Autodesk Inventor part; units mm, degrees
ref_plane "YZ Plane" through (0, 0, 0) normal (1, 0, 0) x (0, 1, 0)
ref_plane "XZ Plane" through (0, 0, 0) normal (0, 1, 0) x (-1, 0, 0)
ref_plane "XY Plane" through (0, 0, 0) normal (0, 0, 1) x (1, 0, 0)
sketch "Sketch1" plane through (0, 0, 0) normal (0, 1, 0) x (-1, 0, 0)
  line L0 (101.6, -101.6) -> (-101.6, -101.6)
  line L1 (-101.6, -101.6) -> (-101.6, 101.6)
  line L2 (-101.6, 101.6) -> (101.6, 101.6)
  line L3 (101.6, 101.6) -> (101.6, -101.6)
  line L4 (96.6, -96.6) -> (-96.6, -96.6)
  line L5 (-96.6, -96.6) -> (-96.6, 96.6)
  line L6 (-96.6, 96.6) -> (96.6, 96.6)
  line L7 (96.6, 96.6) -> (96.6, -96.6)
  line L8 (101.6, 101.6) -> (-40.4, 101.6)
  circle A0 centre (0, 0) radius 88.9
  line L9 (-40.4, 101.6) -> (-101.6, 40.4)
  line L10 (-45.4, 101.6) -> (-101.6, 45.4)
  line L11 (96.6, 96.6) -> (96.6, 101.6)
  line L12 (-45.4, 101.6) -> (-35.4, 101.6)
  line L13 (-35.4, 101.6) -> (-35.4, 96.6)
  line L14 (-35.4, 96.6) -> (-45.4, 96.6)
  line L15 (-45.4, 96.6) -> (-45.4, 101.6)
  line L16 (-101.6, 39.4) -> (-39.4, 101.6)
  line L17 (96.4, -96.4) -> (-96.4, -96.4)
  line L18 (-96.4, -96.4) -> (-96.4, 96.4)
  line L19 (-96.4, 96.4) -> (96.4, 96.4)
  line L20 (96.4, 96.4) -> (96.4, -96.4)
  circle A1 centre (0, 0) radius 90.9
  point P0 (96.6, 51.2168)
  point P1 (101.6, 40.4)
  point P2 (101.6, -40.4)
  point P3 (96.6, -51.2168)
  point P4 (-96.6, 45.4)
  point P5 (-45.4, 96.6)
  point P6 (-44.6, 96.4)
  point P7 (-96.4, 44.6)
  dimension "d0" = 203.2
  dimension "d1" = 203.2
  dimension "d2" = 101.6
  dimension "d3" = 101.6
  dimension "d4" = 5
  dimension "d5" = 5
  dimension "d6" = 5
  dimension "d7" = 5
  dimension "d8" = 142
  dimension "d9" = 61.2
  dimension "d10" = 177.8
  dimension "d11" = 5
  dimension "d12" = 5
  dimension "d13" = 10
  dimension "d14" = 1
  dimension "d15" = 0.2
  dimension "d16" = 0.2
  dimension "d17" = 0.2
  dimension "d18" = 0.2
  dimension "d64" = 181.8
extrude "Extrusion1" add sketch "Sketch1" along normal blind 4 contours L16 L19 L20 L17 L18
sketch "Sketch6" plane through (0, 4, 0) normal (0, 1, 0) x (1, 0, 0)
  line L0 (96.4, 96.4) -> (-96.4, 96.4)
  line L1 (96.4, 96.4) -> (88.4, 96.4)
  line L2 (88.4, 96.4) -> (88.4, -45.6)
  line L3 (88.4, -45.6) -> (96.4, -45.6)
  line L4 (96.4, -45.6) -> (96.4, 96.4)
  line L5 (96.4, -44.6) -> (96.4, 96.4)
  line L6 (88.4, -12) -> (96.4, -12)
  line L7 (96.4, -12) -> (96.4, 12)
  line L8 (96.4, 12) -> (88.4, 12)
  line L9 (88.4, 12) -> (88.4, -12)
  line L10 (0, 0) -> (96.4, 0)
  point P0 (96.4, -12)
  dimension "d58" = 8
  dimension "d59" = 142
  dimension "d62" = 12
  dimension "d63" = 12
extrude "Extrusion6" cut sketch "Sketch6" against normal blind 25.4 contours L4 L10 L2 L8 | L4 L6 L2 L10
sketch "Sketch8" plane through (0, 4, 0) normal (0, 1, 0) x (1, 0, 0)
  line L0 (-96.6, 96.6) -> (-96.6, -96.6)
  line L1 (96.6, 96.6) -> (-96.6, 96.6)
  line L2 (-96.6, 96.6) -> (96.6, 96.6)
  line L3 (96.6, -45.4) -> (45.4, -96.6)
  line L4 (96.6, 96.6) -> (96.6, -45.4)
  line L5 (96.6, -45.4) -> (45.4, -96.6)
  line L6 (45.4, -96.6) -> (-96.6, -96.6)
  line L7 (-96.6, -96.6) -> (-96.6, 96.6)
  line L8 (-96.6, 96.6) -> (-89.5289, 89.5289)
  circle A0 centre (-89.5289, 89.5289) radius 5
  circle A1 centre (-89.5289, 89.5289) radius 1.5
  line L9 (-89.5289, 84.5289) -> (-96.6, 84.5289)
  line L10 (-89.5289, 89.5289) -> (-89.5289, 84.5289)
  line L11 (-89.5289, 89.5289) -> (-84.5289, 89.5289)
  line L12 (-84.5289, 96.6) -> (-84.5289, 89.5289)
  line L13 (-96.6, -96.6) -> (-89.5289, -89.5289)
  line L14 (-96.6, -96.6) -> (-86.6, -96.6) construction
  circle A2 centre (-89.5289, -89.5289) radius 5
  circle A3 centre (-89.5289, -89.5289) radius 1.75
  line L15 (-89.5289, -89.5289) -> (-84.5289, -89.5289)
  line L16 (-84.5289, -96.6) -> (-84.5289, -89.5289)
  line L17 (-89.5289, -89.5289) -> (-89.5289, -84.5289)
  line L18 (-96.6, -84.5289) -> (-89.5289, -84.5289)
  line L19 (96.6, 96.6) -> (89.5289, 89.5289)
  circle A4 centre (89.5289, 89.5289) radius 5
  circle A5 centre (89.5289, 89.5289) radius 1.75
  line L20 (89.5289, 89.5289) -> (84.5289, 89.5289)
  line L21 (84.5289, 96.6) -> (84.5289, 89.5289)
  line L22 (89.5289, 89.5289) -> (89.5289, 84.5289)
  line L23 (96.6, 84.5289) -> (89.5289, 84.5289)
  line L24 (96.6, -43.114) -> (96.6, 96.6)
  line L25 (-96.6, -96.6) -> (43.1178, -96.6)
  line L26 (28.9914, 5.6569) -> (-5.6569, -28.9914)
  line L27 (25.4, -25.4) -> (101.6, -25.4)
  line L28 (101.6, -88.9) -> (101.6, 101.6)
  line L29 (25.4, -25.4) -> (25.4, -101.6)
  line L30 (43.1178, -101.6) -> (-101.6, -101.6)
  line L31 (96.6, -25.4) -> (86.6, -25.4)
  circle A6 centre (86.6, -25.4) radius 5
  circle A7 centre (86.6, -25.4) radius 1.75
  line L32 (25.4, -96.6) -> (25.4, -86.6)
  circle A8 centre (25.4, -86.6) radius 5
  circle A9 centre (25.4, -86.6) radius 1.75
  line L33 (44.6, -96.4) -> (96.4, -44.6)
  circle A10 centre (68.7322, -68.7322) radius 1
  point P0 (0, 0)
  point P1 (0, 0)
  point P2 (0, 0)
  dimension "d90" = 10
  dimension "d91" = 3
  dimension "d92" = 10
  dimension "d93" = 45
  dimension "d94" = 10
  dimension "d95" = 3.5
  dimension "d96" = 10
  dimension "d97" = 10
  dimension "d98" = 3.5
  dimension "d99" = 76.2
  dimension "d100" = 76.2
  dimension "d101" = 10
  dimension "d102" = 10
  dimension "d103" = 3.5
  dimension "d104" = 10
  dimension "d105" = 10
  dimension "d106" = 3.5
  dimension "d115" = 2
  dimension "d116" = 2.5
hole "Hole1" at (-89.5289, 4, -89.5289) at (89.5289, 4, -89.5289) at (-89.5289, 4, 89.5289) at (68.7322, 4, 68.7322) direction (0, -1, 0) diameter 3.1211 depth 3 tip angle 118 countersink diameter 3.2004 countersink angle 82
fillet "Fillet1" radius 3.175 2 edges at (-6.0132, 0, -90.7009) (-6.0132, 0, 90.7009)
sketch "Sketch9" plane through (0, 4, 0) normal (0, 1, 0) x (1, 0, 0)
  arc A0 (-101.6, -98.425) -> (-98.425, -101.6) centre (-98.425, -98.425) ccw
  line L0 (44.0849, 101.6) -> (-98.425, 101.6)
  line L1 (-101.6, 98.425) -> (-101.6, -98.425)
  line L2 (-101.6, -46.1) -> (-101.6, -76.6)
  line L3 (-96.6, -96.6) -> (-96.6, 96.6)
  line L4 (-96.6, -46.1) -> (-96.6, -76.6)
  line L5 (-101.6, -76.6) -> (-96.6, -76.6)
  line L6 (-101.6, -46.1) -> (-96.6, -46.1)
  line L7 (-98.425, -101.6) -> (101.6, -101.6)
  line L8 (0, 0) -> (-101.6, 0)
  line L9 (-101.6, 46.1) -> (-101.6, 76.6)
  line L10 (-96.6, 46.1) -> (-96.6, 76.6)
  line L11 (-101.6, 76.6) -> (-96.6, 76.6)
  line L12 (-101.6, 46.1) -> (-96.6, 46.1)
  line L13 (-96.6, -76.6) -> (-90.1, -76.6)
  line L14 (-90.1, -76.6) -> (-90.1, -46.1)
  line L15 (-90.1, -46.1) -> (-96.6, -46.1)
  line L16 (-96.6, -46.1) -> (-96.6, -76.6)
  arc A1 (-98.425, 101.6) -> (-101.6, 98.425) centre (-98.425, 98.425) ccw
  line L17 (-101.6, 46.1) -> (-96.6, 46.1)
  line L18 (-90.1, 46.1) -> (-96.6, 46.1)
  line L19 (-101.6, 46.1) -> (-101.6, 76.6)
  line L20 (-96.6, 46.1) -> (-96.6, 76.6)
  line L21 (-96.6, 46.1) -> (-96.6, 76.6)
  line L22 (-90.1, 76.6) -> (-90.1, 46.1)
  line L23 (-101.6, 76.6) -> (-96.6, 76.6)
  line L24 (-96.6, 76.6) -> (-90.1, 76.6)
  point P0 (-98.425, 98.425)
  point P1 (46.1, 101.6)
  point P2 (46.1, 96.6)
  point P3 (76.6, 96.6)
  point P4 (76.6, 101.6)
  point P5 (-46.1, 96.6)
  dimension "d117" = 30.5
  dimension "d118" = 25
  dimension "d119" = 6.5
extrude "Extrusion7" cut sketch "Sketch9" against normal blind 25.4 contours L24 L22 L18 L3 | L15 L14 L13 L3
equation "\"d1\" = d0"
equation "\"d15\" = d17"
equation "\"d16\" = d17"
equation "\"d18\" = d17"
properties part number "Drop_Plate"
Check sheet for the modelled part. Datum: model origin and axes. Units: mm. Give positions to 0.01 mm unless a question says otherwise; leave off trailing zeros. Order: outer loops, then holes, each group sorted by start corner. A loop starts at its lowest first (then second) coordinate and runs counter-clockwise, first axis right, second up. Notation, with made-up numbers: (13.25, -18.5) - (51.25, -18.5) arc R11 cw to (51.25, -1.5) - close; hole circle Ø5 at (73, 87.25). An arc over 180 degrees is marked (long way). Answer as CSV lines item,"result".
1. Scan lines: probe 1 along Z at (x, y) = (68.5, 2.7); probe 2 along X at (y, z) = (3.75, 43.5); probe 3 along X at (y, z) = (0.3, -32). Record each from-to range of solid material in increasing order. Write a range as from..to.
Result sheet:
probe 1,"-96.4..-59.81, 59.81..67.19, 70.28..72.5"
probe 2,"-96.4..-79.82, 79.82..96.4"
probe 3,"-96.4..-87.03, 87.03..96.4"
2. Section check A-A (x = 0). Record the boundary of the cut face in (y, z) (3 decimals), then the cut area to 3 significant figures.
Result sheet:
outline,"(0, -96.4) - (4, -96.4) - (4, -90.9) - (3.175, -90.9) arc R3.175 ccw to (0, -94.075) - close; (0, 94.075) arc R3.175 ccw to (3.175, 90.9) - (4, 90.9) - (4, 96.4) - (0, 96.4) - close"
area,"39.7 mm²"
3. Go/stop test with flat-tipped pins: P1, Ø2, axis at y = 2.5, z = 58.5, coming from the -X side; P2, Ø2.5, axis at x = 68.73, z = 68.73, coming from the +Y side; P3, Ø1.9, axis at x = -89.53, z = 89.53, coming from the +Y side. Record where each tip stops, or that it passes through.
Result sheet:
P1,"x = -90.1"
P2,"y = 0.82"
P3,"y = 0.63"
4. Section check B-B (y = 2.1). Record the boundary of the cut face in (x, z).
Result sheet:
outline,"(-96.4, -96.4) - (96.4, -96.4) - (96.4, -12) - (90.29, -12) arc R91.09 cw (long way) to (90.29, 12) - (96.4, 12) - (96.4, 44.6) - (44.6, 96.4) - (-96.4, 96.4) - (-96.4, 76.6) - (-90.1, 76.6) - (-90.1, 46.1) - (-96.4, 46.1) - (-96.4, -46.1) - (-90.1, -46.1) - (-90.1, -76.6) - (-96.4, -76.6) - close; hole circle Ø3.12 at (-89.53, -89.53); hole circle Ø3.12 at (-89.53, 89.53); hole circle Ø3.12 at (68.73, 68.73); hole circle Ø3.12 at (89.53, -89.53)"
5. Mould release check, pull along Z, two halves, no side actions. Record for faces 1 (the face through (-90.82, 3.58, 3.83)), 2 (the face through (71, 2, 70)), 3 (the face through (-92, 4, 0)): released by +Z, released by -Z, zero draft, split by the parting line, or undercut.
Result sheet:
face 1,"undercut"
face 2,"released by +Z"
face 3,"zero draft"
6. Section check C-C (z = 0). Record the boundary of the cut face in (x, y) (3 decimals).
Result sheet:
outline,"(-96.4, 0) - (-94.075, 0) arc R3.175 ccw to (-90.9, 3.175) - (-90.9, 4) - (-96.4, 4) - close"
